Here's how the part is built. I have some questions about the finished solid (model axes, mm). Round coordinates to 2 decimals unless told otherwise and drop trailing zeros. Write each loop counter-clockwise with the first axis right and the second up, starting at its lowest first coordinate (ties: lowest second). Pieces come first, ordered by that corner, then holes. Notation, with made-up numbers: (-25, -3) -> (8, -3) arc R4 ccw to (8, 2) -> close; hole circle Ø1 at (70.5, -31). An arc over 180 degrees is marked (long way). Put each result on its own line as item: value. Start each with the question number.
1. I need wall thicknesses on probe 1 along Y at (x, z) = (-325, 3); probe 2 along X at (y, z) = (-433, 10.5). Which ranges of each line are inside material? Lowest first, please. Write a range as from..to.
2. Suppose I cut it at A-A (x = -377.5). Please give me the cut outline in (y, z), then the cut area to 3 significant figures.
3. Suppose I cut it at B-B (z = 4.25). Count the separate pieces of the cut face and the enclosed holes in it, then the cut area to 3 significant figures.
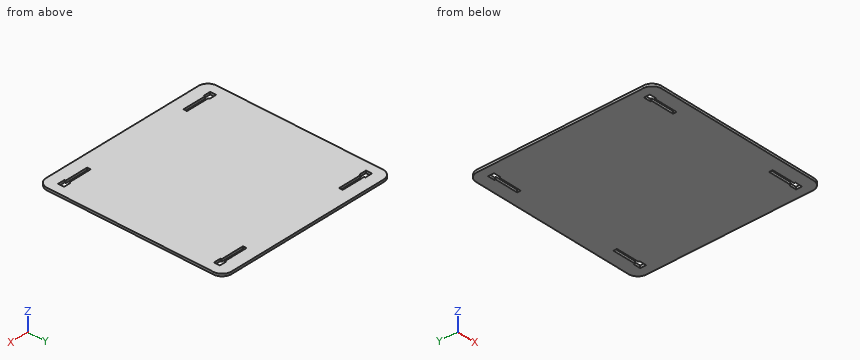
```python
from build123d import *

# Parameters (mm, degrees)
F1_DEPTH = 12.7


with BuildPart() as f1:
    # F0 (on Top) → F1 (new body)
    with BuildSketch(Plane.XY):
        with BuildLine():
            Line((0, 500), (-449.2, 500))
            ThreePointArc((-449.2, 500), (-485.121024, 485.121024), (-500, 449.2))
            Line((-500, 449.2), (-500, 0))
            Line((-500, 0), (0, 0))
            Line((0, 0), (0, 500))
        make_face()
        Polygon((-411.1, 410.973), (-411.1, 404.496), (-449.2, 404.496), (-449.2, 436.5), (-411.1, 436.5), (-411.1, 430.023), (-284.1, 430.023), (-284.1, 410.973), align=None, mode=Mode.SUBTRACT)
        with BuildLine():
            Line((449.2, 500), (0, 500))
            Line((0, 500), (0, 0))
            Line((0, 0), (500, 0))
            Line((500, 0), (500, 449.2))
            ThreePointArc((500, 449.2), (485.121024, 485.121024), (449.2, 500))
        make_face()
        Polygon((411.1, 430.023), (411.1, 436.5), (449.2, 436.5), (449.2, 404.496), (411.1, 404.496), (411.1, 410.973), (284.1, 410.973), (284.1, 430.023), align=None, mode=Mode.SUBTRACT)
        with BuildLine():
            Line((500, 0), (0, 0))
            Line((0, 0), (0, -500))
            Line((0, -500), (449.2, -500))
            ThreePointArc((449.2, -500), (485.121024, -485.121024), (500, -449.2))
            Line((500, -449.2), (500, 0))
        make_face()
        Polygon((284.1, -430.023), (284.1, -410.973), (411.1, -410.973), (411.1, -404.496), (449.2, -404.496), (449.2, -436.5), (411.1, -436.5), (411.1, -430.023), align=None, mode=Mode.SUBTRACT)
        with BuildLine():
            Line((0, -500), (0, 0))
            Line((0, 0), (-500, 0))
            Line((-500, 0), (-500, -449.2))
            ThreePointArc((-500, -449.2), (-485.121024, -485.121024), (-449.2, -500))
            Line((-449.2, -500), (0, -500))
        make_face()
        Polygon((-449.2, -436.5), (-449.2, -404.496), (-411.1, -404.496), (-411.1, -410.973), (-284.1, -410.973), (-284.1, -430.023), (-411.1, -430.023), (-411.1, -436.5), align=None, mode=Mode.SUBTRACT)
    extrude(amount=F1_DEPTH)


solid = f1.part
```
Verdict:
1. probe 1: y = -500..-430.02, -410.97..410.97, 430.02..500
1. probe 2: x = -500..-449.2, -411.1..411.1, 449.2..500
2. outline: (-500, 0) -> (-430.02, 0) -> (-430.02, 12.7) -> (-500, 12.7) -> close; (-410.97, 0) -> (410.97, 0) -> (410.97, 12.7) -> (-410.97, 12.7) -> close; (430.02, 0) -> (500, 0) -> (500, 12.7) -> (430.02, 12.7) -> close
2. area: 12,200 mm^2
3. separate pieces: 1
3. enclosed holes: 4
3. area: 983,000 mm^2
